Input: part model. Units: mm. Frame: model coordinates. A direction names the side the tool comes from. Round coordinates to 2 decimals unless told otherwise and drop trailing zeros. Order: outer loops, then holes, each group sorted by start corner. A loop starts at its lowest first (then second) coordinate and runs counter-clockwise, first axis right, second up. Notation, with made-up numbers: M 16,50 L 40,50 A9 ccw 40,64 Z; hole C 35,-38.75 d4. An arc over 180 degrees is marked long. One line per question, with ' | ' between items.
```python
from build123d import *

# Parameters (mm, degrees)
SKETCH1_W           = 17.792403666
SKETCH1_H           = 18.201033873
SKETCH1_W_2         = 2
BOSS_EXTRUDE1_DEPTH = 2
SKETCH1_3_W         = 2
SKETCH1_3_H         = 18.201033873
BOSS_EXTRUDE2_DEPTH = 13
FILLET1_R           = 3


with BuildPart() as part:
    # Sketch1 → Boss-Extrude1 (new body)
    with BuildSketch(Plane(origin=(0, 0, 0), x_dir=(1, 0, 0), z_dir=(0, 1, 0))):
        with Locations((-0.033894989, -2.255649147)):
            Rectangle(SKETCH1_W, SKETCH1_H)
        with Locations((-9.930096822, -2.255649147)):
            Rectangle(SKETCH1_W_2, SKETCH1_H)
        with Locations((9.862306844, -2.255649147)):
            Rectangle(SKETCH1_W_2, SKETCH1_H)
    extrude(amount=BOSS_EXTRUDE1_DEPTH)

    # Sketch1_3 → Boss-Extrude2 (add)
    with BuildSketch(Plane(origin=(0, 0, 0), x_dir=(1, 0, 0), z_dir=(0, 1, 0))):
        with Locations((-9.930096822, -2.255649147)):
            Rectangle(SKETCH1_3_W, SKETCH1_3_H)
        with Locations((9.862306844, -2.255649147)):
            Rectangle(SKETCH1_3_W, SKETCH1_3_H)
    extrude(amount=BOSS_EXTRUDE2_DEPTH)

    # Fillet1
    fillet1_edges = [part.edges().sort_by_distance(p)[0] for p in [
        (-8.930096822, 2, 2.255649147),
        (8.862306844, 2, 2.255649147),
        (-10.930096822, 0, 2.255649147),
        (10.862306844, 0, 2.255649147),
    ]]
    fillet(fillet1_edges, radius=FILLET1_R)


solid = part.part
```
Item 1: Access query for faces 1 (the flat face through (0.8, 1.7, -6.845)), 2 (the flat face through (8.862, 9, 2)). Directions: +Z, -Z, +X, -X, +Y, -Y. A direction counts if a zero-diameter tool reaches every point of the face in a straight line with its end or side. Return the directions, or none.
Report:
face 1: -Z, +X, -X, +Y, -Y | face 2: +Z, -Z, +Y
Item 2: Section query C-C, the plane y = 3.75. Return loops of the section in (x, z).
Report:
outline: M -10.93,-6.84 L -8.66,-6.84 L -8.66,11.36 L -10.93,11.36 Z; M 8.59,-6.84 L 10.86,-6.84 L 10.86,11.36 L 8.59,11.36 Z
Item 3: Line query: line 1 along X through (y, z) = (6.5, 8.25); line 2 along Y through (x, z) = (6, -1); line 3 along Y through (x, z) = (10, 8). Output: solid intervals per line, ascending. Write a range as from..to.
Report:
line 1: -10.93..-8.93, 8.86..10.86 | line 2: 0..2 | line 3: 0.9..13
Item 4: Section query D-D, the plane x = -3.25. Return loops of the section in (y, z), plus the area to 3 significant figures.
Report:
outline: M 0,-6.84 L 2,-6.84 L 2,11.36 L 0,11.36 Z | area: 36.4 mm²
Item 5: Mould query, pull axis X, two halves, no side actions, for faces 3 (the cylindrical face through (9.96, 0.855, 2.128)), 4 (the cylindrical face through (-10.07, 0.9, 2.13)), 5 (the flat face through (-8.93, 9, 2)). Classes: +X half, -X half, draft (parallel to the pull), parting line (faces both ways), or undercut.
Report:
face 3: +X half | face 4: -X half | face 5: undercut
Item 6: First-contact query: pin 1 (1 mm diameter, centred on x = -8.5, z = 9, fed in from +Y); pin 2 (6 mm diameter, centred on x = -2, z = 5, fed in from +Y). Flat tips, straight axial feed; report the tip coordinate or a pass-through.
Report:
pin 1: y = 13 | pin 2: y = 2
Item 7: Section query A-A, the plane y = 10. Return loops of the section in (x, z), plus the area to 3 significant figures.
Report:
outline: M -10.93,-6.84 L -8.93,-6.84 L -8.93,11.36 L -10.93,11.36 Z; M 8.86,-6.84 L 10.86,-6.84 L 10.86,11.36 L 8.86,11.36 Z | area: 72.8 mm²
Item 8: Section query B-B, the plane z = 3. Return loops of the section in (x, y).
Report:
outline: M -10.93,3 A3 ccw -7.93,0 L 7.86,0 A3 ccw 10.86,3 L 10.86,13 L 8.86,13 L 8.86,5 A3 cw 5.86,2 L -5.93,2 A3 cw -8.93,5 L -8.93,13 L -10.93,13 Z
